The listing builds one solid part. Answer for the finished solid, in the listing's coordinates (mm). A direction names the side the tool comes from. Coordinates: 2 decimals unless noted, no trailing zeros. Write each loop counter-clockwise with the first axis right and the second up, starting at its lowest first coordinate (ties: lowest second). Pieces come first, ordered by that corner, then holes. Notation, with made-up numbers: M -33,64 L 8,64 A33 cw 8,93 Z; hole C -13.75,12 d5. An arc over 180 degrees is marked long. Answer as CSV lines item,"result".
```python
from build123d import *

# Parameters (mm, degrees)
EXTRUDE_1_DEPTH     = 12
CHAMFER_1_SIZE      = 0.2
SKETCH_2_R          = 1.5
CUT_EXTRUDE_1_DEPTH = 27.236731885
CHAMFER_2_SIZE      = 1


with BuildPart() as part:
    # 草图1 → 凸台-拉伸1 (new body)
    with BuildSketch(Plane.XY):
        Polygon((0, 0), (0, 21.31), (9.5, 21.31), (9.5, 16.31), (8.2, 16.31), (8.2, 14.71), (3, 14.71), (3, 5), (9.5, 5), (9.5, 0), align=None)
    extrude(amount=EXTRUDE_1_DEPTH)

    # 倒角1
    chamfer_1_edges = [part.edges().sort_by_distance(p)[0] for p in [
        (8.2, 14.71, 6),
    ]]
    chamfer(chamfer_1_edges, length=CHAMFER_1_SIZE)

    # 草图2 → 切除-拉伸1 (cut, through all)
    with BuildSketch(Plane.ZY):
        with Locations((9, 18.81)):
            Circle(SKETCH_2_R)
        with Locations((3, 18.81)):
            Circle(SKETCH_2_R)
        with Locations((3, 2.5)):
            Circle(SKETCH_2_R)
        with Locations((9, 2.5)):
            Circle(SKETCH_2_R)
    extrude(amount=-CUT_EXTRUDE_1_DEPTH, mode=Mode.SUBTRACT)

    # 倒角2
    chamfer_2_edges = [part.edges().sort_by_distance(p)[0] for p in [
        (0, 0, 6),
        (0, 21.31, 6),
    ]]
    chamfer(chamfer_2_edges, length=CHAMFER_2_SIZE - 0.0001)  # a hair under: the kernel refuses the full size


solid = part.part
```
Q1. Find section A-A (x = 4). Give the vertices of the cut face in (y, z).
Output:
outline,"M 0,0 L 5,0 L 5,12 L 0,12 Z; M 14.71,0 L 21.31,0 L 21.31,12 L 14.71,12 Z; hole C 2.5,3 d3; hole C 2.5,9 d3; hole C 18.81,3 d3; hole C 18.81,9 d3"
Q2. Find section D-D (z = 9). Count the separate pieces of the cut face and the enclosed holes in it, and give its area (3 significant figures).
Output:
separate pieces,"3"
enclosed holes,"0"
area,"79.2 mm2"
Q3. Straight lines are drawn through the part: line 1 (Y direction, x = 4.75, z = 4.75); line 2 (Y direction, x = 5.5, z = 2.75); line 3 (Z direction, x = 7, y = 19.5). For each, find the intervals that lie inside material, in ascending order.
Output:
line 1,"0 to 5, 14.71 to 21.31"
line 2,"0 to 1.02, 3.98 to 5, 14.71 to 17.33, 20.29 to 21.31"
line 3,"0 to 1.67, 4.33 to 7.67, 10.33 to 12"
Q4. Flat-ended cylindrical pins translate along their axes: pin 1 Ø5 at (y, z) = (11.5, 9) entering from +X; pin 2 Ø1.8 at (y, z) = (18.81, 3) entering from +X. Find the tip coordinate at first contact, or state that the pin passes through.
Output:
pin 1,"x = 3"
pin 2,"through"
Q5. Find section C-C (y = 18.81). Give the vertices of the cut face in (x, z), and give its area (3 significant figures).
Output:
outline,"M 0,0 L 9.5,0 L 9.5,1.5 L 0,1.5 Z; M 0,4.5 L 9.5,4.5 L 9.5,7.5 L 0,7.5 Z; M 0,10.5 L 9.5,10.5 L 9.5,12 L 0,12 Z"
area,"57.0 mm2"
Q6. Find section B-B (x = 2). Give the vertices of the cut face in (y, z), and give its area (3 significant figures).
Output:
outline,"M 0,0 L 21.31,0 L 21.31,12 L 0,12 Z; hole C 2.5,3 d3; hole C 2.5,9 d3; hole C 18.81,3 d3; hole C 18.81,9 d3"
area,"227 mm2"
Q7. For faces 1 (the flat face through (9.5, 3, 6)), 2 (the flat face through (9, 16.31, 6)), determine the directions among +Z, -Z, +X, -X, +Y, -Y from which every point of the face is accessible in a straight line to the end or side of a thin tool.
Output:
face 1,"+Z, -Z, +X, +Y, -Y"
face 2,"+Z, -Z, +X"
Q8. The mould has two halves that part along Z. Classify faces 3 (the flat face through (2.7, 10.8, 12)), 4 (the cylindrical face through (4.68, 1.17, 3.69)), 5 (the flat face through (0, 11, 6)), 6 (the flat face through (2.7, 10.8, 0)): pulls with the +Z half, pulls with the -Z half, needs draft (parallel to the pull), parting line crosses it, or undercut.
Output:
face 3,"pulls with the +Z half"
face 4,"undercut"
face 5,"needs draft"
face 6,"pulls with the -Z half"
